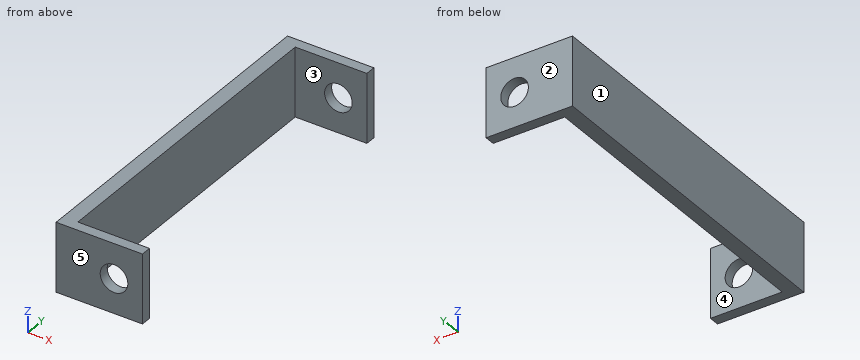
```python
from build123d import *

# Parameters (mm, degrees)
SKETCH1_W           = 25
SKETCH1_H           = 20
SKETCH1_R           = 4
BOSS_EXTRUDE1_DEPTH = 3
SKETCH2_W           = 4.260066628
SKETCH2_H           = 20
BOSS_EXTRUDE2_DEPTH = 93.06
SKETCH3_W           = 25
SKETCH3_H           = 20
SKETCH3_R           = 4
BOSS_EXTRUDE3_DEPTH = 3


with BuildPart() as part:
    # Sketch1 → Boss-Extrude1 (new body)
    with BuildSketch(Plane(origin=(0, 0, 0), x_dir=(1, 0, 0), z_dir=(0, 1, 0))):
        with Locations((12.5, 10)):
            Rectangle(SKETCH1_W, SKETCH1_H)
        with Locations(Location((16.760066628, 10, 0), (0, 0, 270))):
            Circle(SKETCH1_R, mode=Mode.SUBTRACT)
    extrude(amount=BOSS_EXTRUDE1_DEPTH)

    # Sketch2 → Boss-Extrude2 (add)
    with BuildSketch(Plane(origin=(0, 3, 0), x_dir=(1, 0, 0), z_dir=(0, 1, 0))):
        with Locations((2.130033314, 10)):
            Rectangle(SKETCH2_W, SKETCH2_H)
    extrude(amount=BOSS_EXTRUDE2_DEPTH)

    # Sketch3 → Boss-Extrude3 (add)
    with BuildSketch(Plane(origin=(0, 96.06, 0), x_dir=(1, 0, 0), z_dir=(0, 1, 0))):
        with Locations((12.5, 10)):
            Rectangle(SKETCH3_W, SKETCH3_H)
        with Locations(Location((16.760066628, 10, 0), (0, 0, 270))):
            Circle(SKETCH3_R, mode=Mode.SUBTRACT)
    extrude(amount=BOSS_EXTRUDE3_DEPTH)


solid = part.part
```
Model file for the job. Use its own axes, mm. Face numbers are marked on the shaded views. A direction names the side the tool comes from. Coordinates: 2 decimals unless noted, no trailing zeros. Order: outer loops, then holes, each group sorted by start corner. A loop starts at its lowest first (then second) coordinate and runs counter-clockwise, first axis right, second up. Notation, with made-up numbers: (4, 31) -> (34, 31) arc R29 cw to (34, 55) -> close; hole circle Ø1 at (7, 20.5). An arc over 180 degrees is marked (long way). Answer as a JSON object with one key per item and string values. Group by question number.
1) Cut at B-B, the plane z = -10. Write the cut outline in (x, y), then the cut area to 3 significant figures.
2) Pull direction Y, two halves, no side cores. Call the marked faces 1, 2 and 3: +Y half, -Y half, draft (parallel to the pull), parting line (faces both ways), or undercut.
3) Cut at D-D, the plane x = 18.25. Write the cut outline in (y, z), then the cut area to 3 significant figures.
4) Flat gauge pin, fed straight in: pin 1 (10 mm diameter, centred on y = 41, z = -6.5, fed in from +X). Where does the tip first touch, or does it go through?
5) Which spindle directions (+Z, -Z, +X, -X, +Y, -Y) get a long thin tool onto all of the face, cutting with end or side? Do the marked faces 4 and 5. Say none if no direction does.
6) Cut at C-C, the plane z = -4.5. Write the cut outline in (x, y), then the cut area to 3 significant figures.
7) Drill centre lines: L1, parallel to Y at x = 22.25, z = -11.25; L2, parallel to X at y = 1.05, z = -10; L3, parallel to X at y = 87, z = -2.75. Where is each one in solid material? Low to high.
8) Cut at A-A, the plane x = 10.75. Write the cut outline in (y, z), then the cut area to 3 significant figures.
Check values:
{
 "1": {"outline": "(0, 0) -> (12.76, 0) -> (12.76, 3) -> (4.26, 3) -> (4.26, 96.06) -> (12.76, 96.06) -> (12.76, 99.06) -> (0, 99.06) -> close; (20.76, 0) -> (25, 0) -> (25, 3) -> (20.76, 3) -> close; (20.76, 96.06) -> (25, 96.06) -> (25, 99.06) -> (20.76, 99.06) -> close", "area": "498 mm²"},
 "2": {"face 1": "draft", "face 2": "+Y half", "face 3": "undercut"},
 "3": {"outline": "(0, -20) -> (3, -20) -> (3, -13.71) -> (0, -13.71) -> close; (0, -6.29) -> (3, -6.29) -> (3, 0) -> (0, 0) -> close; (96.06, -20) -> (99.06, -20) -> (99.06, -13.71) -> (96.06, -13.71) -> close; (96.06, -6.29) -> (99.06, -6.29) -> (99.06, 0) -> (96.06, 0) -> close", "area": "75.5 mm²"},
 "4": {"pin 1": "stops at x = 4.26"},
 "5": {"face 4": "+Z, -Z, +X", "face 5": "+Z, -Z, +X, -X, -Y"},
 "6": {"outline": "(0, 0) -> (25, 0) -> (25, 3) -> (4.26, 3) -> (4.26, 96.06) -> (25, 96.06) -> (25, 99.06) -> (0, 99.06) -> close", "area": "546 mm²"},
 "7": {"L1": "y = 0 to 3, 96.06 to 99.06", "L2": "x = 0 to 12.76, 20.76 to 25", "L3": "x = 0 to 4.26"},
 "8": {"outline": "(0, -20) -> (3, -20) -> (3, 0) -> (0, 0) -> close; (96.06, -20) -> (99.06, -20) -> (99.06, 0) -> (96.06, 0) -> close", "area": "120 mm²"}
}
